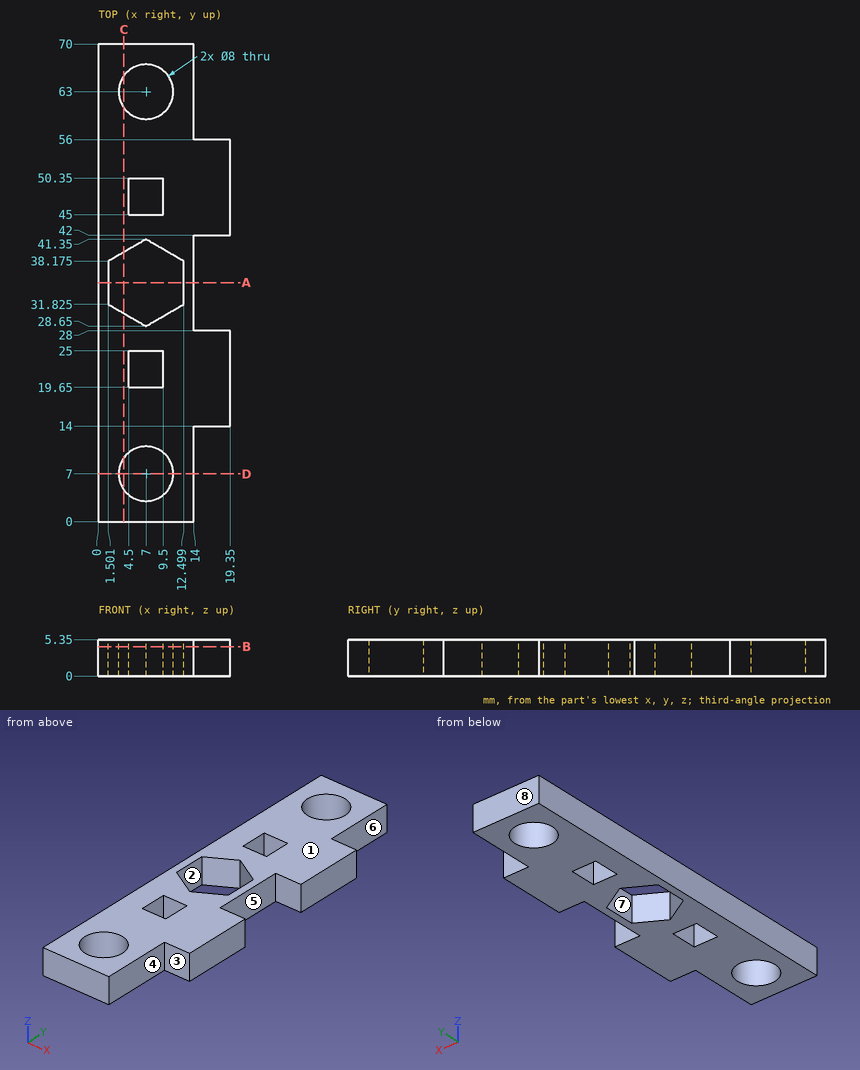
Verification items for this drawing (mm, ordinates from the low corner). A direction names the side the tool comes from. Coordinates: 2 decimals unless noted, no trailing zeros. Write each loop counter-clockwise with the first axis right and the second up, starting at its lowest first coordinate (ties: lowest second). Pieces come first, ordered by that corner, then holes. Notation, with made-up numbers: M -19.5,-32.5 L -7.5,-32.5 A17 cw -7.5,-12.5 Z; hole C 83.5,84.25 d5. An arc over 180 degrees is marked long. Answer as a JSON object with one key per item and string values.
1. Go/stop test with a flat-tipped pin: pin 1 Ø2.5 at (y, z) = (35.5, 4) entering from +X. Record where the tip stops, or that it passes through.
Answers below:
{"pin 1": "stops at x = 14"}
2. Section check B-B, the plane z = 4.3. Give the number of separate pieces and of enclosed holes in the cut face, plus the area to 3 significant figures.
Answers below:
{"separate pieces": "1", "enclosed holes": "5", "area": "871 mm²"}
3. Scan lines: L1, parallel to Y at x = 7, z = 2.65; L2, parallel to X at y = 20, z = 4.9; L3, parallel to X at y = 67.5, z = 2.35. Record each from-to range of solid material in increasing order.
Answers below:
{"L1": "y = 0 to 3, 11 to 19.65, 25 to 28.65, 41.35 to 45, 50.35 to 59, 67 to 70", "L2": "x = 0 to 4.5, 9.5 to 19.35", "L3": "x = 0 to 14"}
4. Section check A-A, the plane y = 35. Enter the section's corners in (x, z).
Answers below:
{"outline": "M 0,0 L 1.5,0 L 1.5,5.35 L 0,5.35 Z; M 12.5,0 L 14,0 L 14,5.35 L 12.5,5.35 Z"}
5. Section check C-C, the plane x = 3.75. Enter the section's corners in (y, z).
Answers below:
{"outline": "M 0,0 L 4.67,0 L 4.67,5.35 L 0,5.35 Z; M 9.33,0 L 30.53,0 L 30.53,5.35 L 9.33,5.35 Z; M 39.47,0 L 60.67,0 L 60.67,5.35 L 39.47,5.35 Z; M 65.33,0 L 70,0 L 70,5.35 L 65.33,5.35 Z"}
6. Section check D-D, the plane y = 7. Enter the section's corners in (x, z).
Answers below:
{"outline": "M 0,0 L 3,0 L 3,5.35 L 0,5.35 Z; M 11,0 L 14,0 L 14,5.35 L 11,5.35 Z"}
7. Draft check along Y on the marked faces 1, 2 and 3. Enter one of: released by +Y, released by -Y, zero draft, split by the parting line, or undercut.
Answers below:
{"face 1": "zero draft", "face 2": "undercut", "face 3": "released by -Y"}
8. Tool access check on the marked faces 4, 5, 6, 7 and 8. Record the directions out of +Z, -Z, +X, -X, +Y, -Y that give a thin tool (end or side, any length) a straight path to the whole face; none if there is none.
Answers below:
{"face 4": "+Z, -Z, +X, -Y", "face 5": "+Z, -Z, +X", "face 6": "+Z, -Z, +X, +Y", "face 7": "+Z, -Z", "face 8": "+Z, -Z, +X, -X, +Y"}
